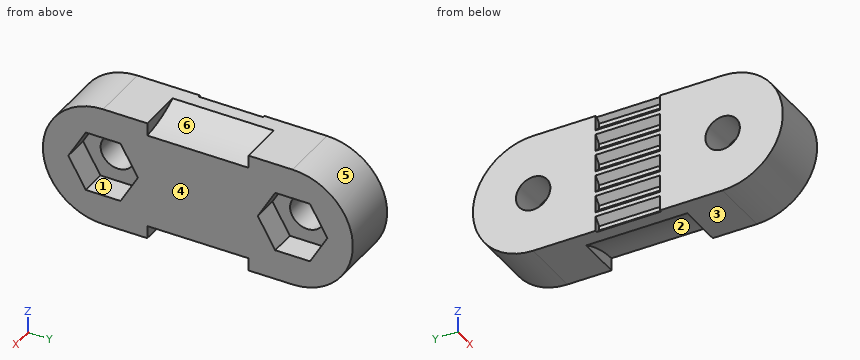
```python
from build123d import *

# Parameters (mm, degrees)
SKETCH019_R         = 1.6
PAD007_DEPTH        = 5.6
POCKET007_DEPTH     = 2.4
POCKET008_DEPTH     = 4.7
POCKET009_DEPTH     = 3
LINEARPATTERN_COUNT = 6
LINEARPATTERN_PITCH = 2


with BuildPart() as part:
    # Sketch019 (on Face6 of Binder001) → Pad007 (new body)
    with BuildSketch(Plane.YZ.offset(-86.1)):
        with BuildLine():
            Line((8.8, 180.6), (-8.8, 180.6))
            ThreePointArc((-8.8, 180.6), (-14.4, 175), (-8.8, 169.4))
            Line((-8.8, 169.4), (8.8, 169.4))
            ThreePointArc((8.8, 169.4), (14.4, 175), (8.8, 180.6))
        make_face()
        with Locations((-8.8, 175)):
            Circle(SKETCH019_R, mode=Mode.SUBTRACT)
        with Locations((8.8, 175)):
            Circle(SKETCH019_R, mode=Mode.SUBTRACT)
    extrude(amount=PAD007_DEPTH)

    # Sketch020 (on Face8 of Pad007) → Pocket007 (cut)
    with BuildSketch(Plane.YZ.offset(-80.5)):
        Polygon((-5.566838, 175), (-7.183419, 177.8), (-10.416581, 177.8), (-12.033162, 175), (-10.416581, 172.2), (-7.183419, 172.2), align=None)
        Polygon((5.566838, 175), (7.183419, 172.2), (10.416581, 172.2), (12.033162, 175), (10.416581, 177.8), (7.183419, 177.8), align=None)
    extrude(amount=-POCKET007_DEPTH, mode=Mode.SUBTRACT)

    # Sketch021 → Pocket008 (cut, symmetric)
    with BuildSketch(Plane.XZ):
        with BuildLine():
            ThreePointArc((-86.9, 182.325421), (-83.976243, 180.26218), (-80.5, 179.41303))
            Line((-80.5, 182.325421), (-80.5, 179.41303))
            Line((-86.9, 182.325421), (-80.5, 182.325421))
        make_face()
        with BuildLine():
            ThreePointArc((-80.5, 170.58697), (-83.976243, 169.73782), (-86.9, 167.674579))
            Line((-86.9, 167.674579), (-80.5, 167.674579))
            Line((-80.5, 167.674579), (-80.5, 170.58697))
        make_face()
    extrude(amount=POCKET008_DEPTH, both=True, mode=Mode.SUBTRACT)

    # Sketch022 → Pocket009 (cut, symmetric)
    with BuildSketch(Plane.XZ):
        Polygon((-86.1, 180.8), (-85.5, 180.2), (-85.5, 179.8), (-86.1, 179.2), align=None)
    pocket009 = extrude(amount=POCKET009_DEPTH, both=True, mode=Mode.SUBTRACT)

    # LinearPattern: Pocket009 ×6
    with Locations(*[(0, 0, -i * LINEARPATTERN_PITCH) for i in range(1, LINEARPATTERN_COUNT)]):
        add(pocket009, mode=Mode.SUBTRACT)


solid = part.part
```
Could you check a few things on this model? Use its own coordinates, in mm. Face numbers are marked on the shaded views. A direction names the side the tool comes from. Coordinates: 2 decimals unless noted, no trailing zeros. Order: outer loops, then holes, each group sorted by start corner. A loop starts at its lowest first (then second) coordinate and runs counter-clockwise, first axis right, second up. Notation, with made-up numbers: M 1,-26.5 L 31,-26.5 A18 cw 31,2.5 Z; hole C -6.75,66.25 d6. An arc over 180 degrees is marked long. Use a Markdown table: item, result. Add a question column.
Q1. I want a section at A-A on y = 9.5. List the corners of the cut face in (x, z) for me, then the cut area to 3 significant figures.
Q2. We'd pull the mould along Y, two halves only. Please class the marked faces 4, 5 and 6: pulls with the +Y half, pulls with the -Y half, needs draft (parallel to the pull), parting line crosses it, or undercut.
Q3. I'm going to push flat-ended pins straight in: pin 1 (0.5 mm diameter, centred on x = -86, z = 180, fed in from +Y); pin 2 (1.3 mm diameter, centred on x = -82, z = 180.5, fed in from +Y); pin 3 (2 mm diameter, centred on x = -82.5, z = 179.5, fed in from +Y). Where does each tip first touch, or does it pass through?
Q4. Which directions (+Z, -Z, +X, -X, +Y, -Y) give clear straight access to the entire face, cutting with the end or side of a thin tool? Please do the marked faces 1, 2 and 3.
Q5. I want a section at D-D on y = -6.75. List the corners of the cut face in (x, z) for me.
Q6. If I drill on L1, parallel to Y at x = -84.35, z = 175; L2, parallel to Z at x = -82.1, y = -8.75; L3, parallel to Z at x = -84.8, y = 8.8, over which ranges is the centre line in solid material (lowest first)?
Q7. I want a section at B-B on y = 1.5. List the corners of the cut face in (x, z) for me.
Q8. I want a section at C-C on x = -84.2. List the corners of the cut face in (y, z) for me, then the cut area to 3 significant figures.
Checked values:
| question | item | result |
|---|---|---|
| 1 | outline | M -86.1,169.44 L -80.5,169.44 L -80.5,172.2 L -82.9,172.2 L -82.9,173.56 L -86.1,173.56 Z; M -86.1,176.44 L -82.9,176.44 L -82.9,177.8 L -80.5,177.8 L -80.5,180.56 L -86.1,180.56 Z |
| 1 | area | 39.6 mm² |
| 2 | face 4 | needs draft |
| 2 | face 5 | pulls with the +Y half |
| 2 | face 6 | undercut |
| 3 | pin 1 | y = 11.77 |
| 3 | pin 2 | y = 11.6 |
| 3 | pin 3 | y = 13.17 |
| 4 | face 1 | +X |
| 4 | face 2 | -Z, +X |
| 4 | face 3 | -Z, +X, -X, +Y, -Y |
| 5 | outline | M -86.1,169.4 L -80.5,169.4 L -80.5,172.95 L -82.9,172.95 L -82.9,177.05 L -80.5,177.05 L -80.5,180.6 L -86.1,180.6 Z |
| 6 | L1 | -14.4 to -10.4, -7.2 to 7.2, 10.4 to 14.4 |
| 6 | L2 | 169.4 to 172.2, 177.8 to 180.6 |
| 6 | L3 | 169.4 to 173.4, 176.6 to 180.6 |
| 7 | outline | M -86.1,170.8 L -85.5,170.2 L -85.5,169.8 L -85.9,169.4 L -84.65,169.4 A9.6 cw -80.5,170.59 L -80.5,179.41 A9.6 cw -84.65,180.6 L -85.9,180.6 L -85.5,180.2 L -85.5,179.8 L -86.1,179.2 L -86.1,178.8 L -85.5,178.2 L -85.5,177.8 L -86.1,177.2 L -86.1,176.8 L -85.5,176.2 L -85.5,175.8 L -86.1,175.2 L -86.1,174.8 L -85.5,174.2 L -85.5,173.8 L -86.1,173.2 L -86.1,172.8 L -85.5,172.2 L -85.5,171.8 L -86.1,171.2 Z |
| 8 | outline | M -8.8,169.4 L -4.7,169.4 L -4.7,169.63 L 4.7,169.63 L 4.7,169.4 L 8.8,169.4 A5.6 ccw 8.8,180.6 L 4.7,180.6 L 4.7,180.37 L -4.7,180.37 L -4.7,180.6 L -8.8,180.6 A5.6 ccw Z; hole C -8.8,175 d3.2; hole C 8.8,175 d3.2 |
| 8 | area | 275 mm² |
